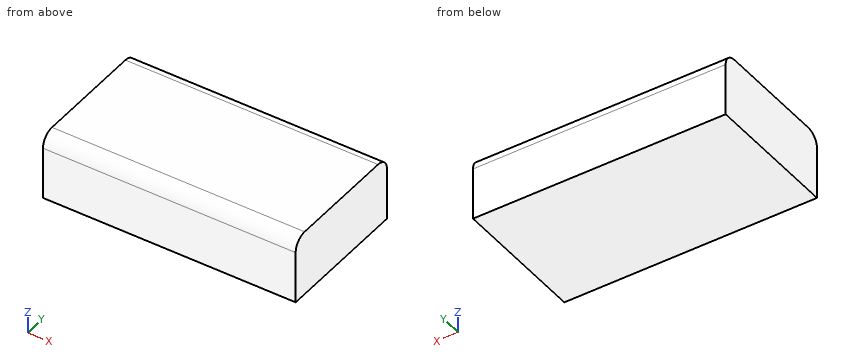
Autodesk Inventor part; units mm, degrees
ref_plane "YZ Plane" through (0, 0, 0) normal (1, 0, 0) x (0, 1, 0)
ref_plane "XZ Plane" through (0, 0, 0) normal (0, 1, 0) x (-1, 0, 0)
ref_plane "XY Plane" through (0, 0, 0) normal (0, 0, 1) x (1, 0, 0)
sketch "Náčrt1" plane through (0, 0, 0) normal (0, 0, 1) x (1, 0, 0)
  line L0 (0, 28.56) -> (0, -28.56)
  line L1 (-53.06, 0) -> (53.06, 0)
  line L2 (-37.9, 20.4) -> (37.9, 20.4)
  line L3 (37.9, 20.4) -> (37.9, -20.4)
  line L4 (37.9, -20.4) -> (-37.9, -20.4)
  line L5 (-37.9, -20.4) -> (-37.9, 20.4)
  point P0 (0, 0)
  dimension "d0" = 75.8
  dimension "d1" = 40.8
extrude "Vysunutí1" add sketch "Náčrt1" along normal blind 19.7
fillet "Zaoblení1" radius 4 2 edges at (0, 20.4, 19.7) (0, -20.4, 19.7)
properties part number "prop_battery"
Verification items for the finished model (mm, model axes). Coordinates: 2 decimals unless noted, no trailing zeros. Order: outer loops, then holes, each group sorted by start corner. A loop starts at its lowest first (then second) coordinate and runs counter-clockwise, first axis right, second up. Notation, with made-up numbers: M -11.75,42.25 L -5.75,42.25 A23 ccw -5.75,65.25 Z; hole C 44.25,-28.5 d11. An arc over 180 degrees is marked long. One line per item, written item: value. Start each with the question number.
Item 1: Sectioned sample at A-A (z = 17.5). Enter the section's corners in (x, y), then the cut area to 3 significant figures.
Item 2: Gauge pin test, flat end, axial feed: pin 1 (1.5 mm diameter, centred on x = 14, y = 12, fed in from -Z). Record the tip position at first contact, or that the pin passes through.
Item 3: Scan lines: probe 1 along Z at (x, y) = (2.5, 18.5); probe 2 along Z at (x, y) = (-29, 17.5); probe 3 along Y at (x, z) = (13.5, 19). Record each from-to range of solid material in increasing order.
Conclusion:
1. outline: M -37.9,-19.97 L 37.9,-19.97 L 37.9,19.97 L -37.9,19.97 Z
1. area: 3,030 mm^2
2. pin 1: stops at z = 0
3. probe 1: z = 0 to 19.1
3. probe 2: z = 0 to 19.55
3. probe 3: y = -18.66 to 18.66
